Part model, mm, in its own coordinate system. Face numbers are marked on the shaded views. Give positions to 0.01 mm unless a question says otherwise; leave off trailing zeros. Order: outer loops, then holes, each group sorted by start corner. A loop starts at its lowest first (then second) coordinate and runs counter-clockwise, first axis right, second up. Notation, with made-up numbers: M 59,24.5 L 96,24.5 A16 ccw 96,39.5 Z; hole C -10,86 d7. An arc over 180 degrees is marked long. Return JSON: item names as keys, results as strings.
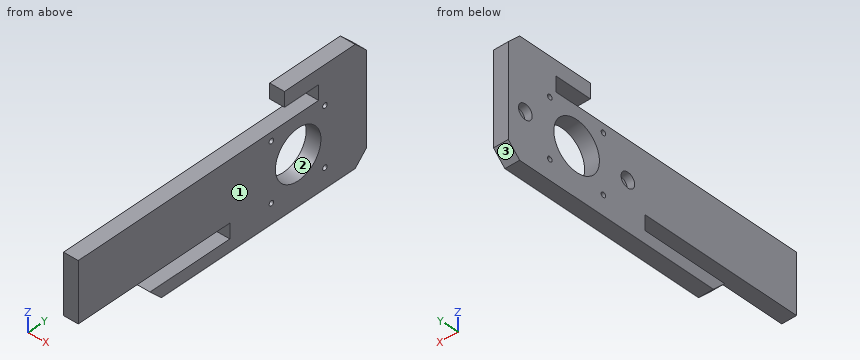
from build123d import *

# Parameters (mm, degrees)
SKETCH1_W                = 59
SKETCH1_H                = 120
SKETCH1_R                = 20
BOSS_EXTRUDE1_DEPTH      = 12
F_4_0_4_DIAMETER_HOLE1_D = 4
HOLE1_D                  = 12
HOLE1_DEPTH              = 6
BOSS_EXTRUDE2_DEPTH      = 12
SKETCH9_W                = 48
SKETCH9_H                = 133
BOSS_EXTRUDE3_DEPTH      = 12
SKETCH11_W               = 10
SKETCH11_H               = 190
BOSS_EXTRUDE4_DEPTH      = 12
CHAMFER1_SIZE            = 10
CHAMFER2_SIZE            = 10


with BuildPart() as part:
    # Sketch1 → Boss-Extrude1 (new body)
    with BuildSketch(Plane(origin=(0, 0, 0), x_dir=(0, 0, -1), z_dir=(1, 0, 0))):
        Rectangle(SKETCH1_W, SKETCH1_H)
        Circle(SKETCH1_R, mode=Mode.SUBTRACT)
    extrude(amount=BOSS_EXTRUDE1_DEPTH)

    # Ø4.0 (4) Diameter Hole1 (through all)
    with Locations(Plane.ZY):
        with Locations((-23.5, 23.5), (23.5, 23.5), (23.5, -23.5), (-23.5, -23.5)):
            Hole(F_4_0_4_DIAMETER_HOLE1_D / 2)

    # Hole1
    with Locations(Plane.ZY):
        with Locations((0, 45), (0, -45)):
            Hole(HOLE1_D / 2, depth=HOLE1_DEPTH)

    # Sketch8 → Boss-Extrude2 (add)
    with BuildSketch(Plane.ZY):
        Polygon((29.5, 60), (29.5, -60), (30.5, -60), (30.5, 18), (42.5, 18), (42.5, -12), (54.5, -12), (54.5, 60), align=None)
    extrude(amount=-BOSS_EXTRUDE2_DEPTH)

    # Sketch9 → Boss-Extrude3 (add)
    with BuildSketch(Plane.ZY):
        with Locations((6.5, -126.5)):
            Rectangle(SKETCH9_W, SKETCH9_H)
    extrude(amount=-BOSS_EXTRUDE3_DEPTH)

    # Sketch11 → Boss-Extrude4 (add)
    with BuildSketch(Plane(origin=(12, 0, 0), x_dir=(0, 0, -1), z_dir=(1, 0, 0))):
        with Locations((34.5, -35)):
            Rectangle(SKETCH11_W, SKETCH11_H)
    extrude(amount=-BOSS_EXTRUDE4_DEPTH)

    # Chamfer1
    chamfer1_edges = [part.edges().sort_by_distance(p)[0] for p in [
        (6, 60, 54.5),
        (6, 60, -39.5),
    ]]
    chamfer(chamfer1_edges, length=CHAMFER1_SIZE)

    # Chamfer2
    chamfer2_edges = [part.edges().sort_by_distance(p)[0] for p in [
        (6, -130, -39.5),
    ]]
    chamfer(chamfer2_edges, length=CHAMFER2_SIZE - 0.0001)  # a hair under: the kernel refuses the full size


solid = part.part
Q1. Band-saw the part on D-D (y = -89). Give the cut face in (x, z), then the cut area to 3 significant figures.
Established:
{"outline": "M 0,-39.5 L 12,-39.5 L 12,-29.5 L 0,-29.5 Z; M 0,-17.5 L 12,-17.5 L 12,30.5 L 0,30.5 Z", "area": "696 mm²"}
Q2. Two-plate mould, pull along Y, no slides. Class the marked faces 1, 2 and 3: +Y half, -Y half, draft (parallel to the pull), parting line (faces both ways), or undercut.
Established:
{"face 1": "draft", "face 2": "undercut", "face 3": "+Y half"}
Q3. Band-saw the part on C-C (x = 2). Give the number of separate pieces and of enclosed holes in the cut face, then the cut area to 3 significant figures.
Established:
{"separate pieces": "1", "enclosed holes": "7", "area": "15,200 mm²"}
Q4. Band-saw the part on A-A (y = 0). Give the cut face in (x, z).
Established:
{"outline": "M 0,-39.5 L 12,-39.5 L 12,-20 L 0,-20 Z; M 0,20 L 12,20 L 12,30.5 L 0,30.5 Z; M 0,42.5 L 12,42.5 L 12,54.5 L 0,54.5 Z"}
Q5. Probe line 1 along Y through (x, z) = (9, -23.5); line 2 along Y through (x, z) = (5.75, 0); line 3 along Z through (x, y) = (3, 23). List the from-to ranges inside material, lowest first.
Established:
{"line 1": "y = -60 to -25.5, -21.5 to 21.5, 25.5 to 60", "line 2": "y = -193 to -51, -39 to -20, 20 to 39, 51 to 60", "line 3": "z = -39.5 to -25.44, -21.56 to 21.56, 25.44 to 54.5"}
Q6. Band-saw the part on B-B (z = 0). Give the cut face in (x, y), then the cut area to 3 significant figures.
Established:
{"outline": "M 0,-193 L 12,-193 L 12,-20 L 0,-20 L 0,-39 L 6,-39 L 6,-51 L 0,-51 Z; M 0,20 L 12,20 L 12,60 L 0,60 L 0,51 L 6,51 L 6,39 L 0,39 Z", "area": "2,410 mm²"}
Q7. Pin check, flat tips, straight feed: pin 1 (3.5 mm diameter, centred on y = 23.5, z = 23.5, fed in from -X); pin 2 (3 mm diameter, centred on x = 9, y = -97.5, fed in from +Z); pin 3 (3.5 mm diameter, centred on x = 4, z = 49, fed in from -Y); pin 4 (11 mm diameter, centred on y = 45, z = 0, fed in from -X). Stop position of each tip, or through.
Established:
{"pin 1": "passes through", "pin 2": "stops at z = 30.5", "pin 3": "stops at y = -12", "pin 4": "stops at x = 6"}
